Build history of the part. All positions in model axes, mm. Coordinates: 2 decimals unless noted, no trailing zeros. Loops run counter-clockwise (first coordinate to the right, second up) from the corner with the lowest first, then second, coordinate; pieces in that order, holes last. Notation, with made-up numbers: (84, -3) - (99, -3) arc R17 cw to (99, 4) - close; hole circle Ø4 at (62, 82.25). An arc over 180 degrees is marked (long way). One line per item, written item: value.
```python
from build123d import *

# Parameters (mm, degrees)
F1_DEPTH = 20
F2_DEPTH = 12
F3_DEPTH = 2
F4_D     = 3.3


with BuildPart() as f1:
    # F0 (on Top) → F1 (new body)
    with BuildSketch(Plane.XY):
        with BuildLine():
            Line((0, 0), (0, 5))
            ThreePointArc((0, 5), (-3.5355339059, -3.5355339059), (5, 0))
            Line((5, 0), (0, 0))
        make_face()
        with BuildLine():
            Line((0, 0), (5, 0))
            ThreePointArc((5, 0), (4.6193976626, 1.9134171618), (3.5355339059, 3.5355339059))
            Line((3.5355339059, 3.5355339059), (0, 0))
        make_face()
        with BuildLine():
            ThreePointArc((3.5355339059, 3.5355339059), (1.9134171618, 4.6193976626), (0, 5))
            Line((0, 5), (0, 0))
            Line((0, 0), (3.5355339059, 3.5355339059))
        make_face()
    extrude(amount=F1_DEPTH)

    # F0 (on Top) → F2 (join)
    with BuildSketch(Plane.XY):
        with BuildLine():
            Line((24.7487373415, 29.7487373415), (0, 5))
            ThreePointArc((0, 5), (1.9134171618, 4.6193976626), (3.5355339059, 3.5355339059))
            ThreePointArc((3.5355339059, 3.5355339059), (4.6193976626, 1.9134171618), (5, 0))
            Line((5, 0), (29.7487373415, 24.7487373415))
            Line((29.7487373415, 24.7487373415), (24.7487373415, 29.7487373415))
        make_face()
    extrude(amount=F2_DEPTH)

    # F0 (on Top) → F3 (cut)
    with BuildSketch(Plane.XY):
        with BuildLine():
            Line((24.7487373415, 29.7487373415), (0, 5))
            ThreePointArc((0, 5), (1.9134171618, 4.6193976626), (3.5355339059, 3.5355339059))
            ThreePointArc((3.5355339059, 3.5355339059), (4.6193976626, 1.9134171618), (5, 0))
            Line((5, 0), (29.7487373415, 24.7487373415))
            Line((29.7487373415, 24.7487373415), (24.7487373415, 29.7487373415))
        make_face()
    extrude(amount=F3_DEPTH, mode=Mode.SUBTRACT)

    # F4 (through all)
    with Locations(Plane(origin=(0, 0, 0), x_dir=(1, 0, 0), z_dir=(0, 0, -1))):
        with Locations((0, 0)):
            Hole(F4_D / 2)


solid = f1.part
```
Item 1: Cut at D-D, the plane x = 15. Write the cut outline in (y, z), then the cut area to 3 significant figures.
Check result:
outline: (10, 2) - (20, 2) - (20, 12) - (10, 12) - close
area: 100 mm^2
Item 2: Probe probe 1 along Y at (x, z) = (0, 8.5); probe 2 along Z at (x, y) = (9.5, 8); probe 3 along X at (y, z) = (1, 10.5). List the from-to ranges inside material, lowest first. Write a range as from..to.
Check result:
probe 1: y = -5..-1.65, 1.65..5
probe 2: z = 2..12
probe 3: x = -4.9..-1.31, 1.31..6
Item 3: Cut at C-C, the plane y = 4. Write the cut outline in (x, z).
Check result:
outline: (-3, 0) - (3, 0) - (3, 2) - (9, 2) - (9, 12) - (3, 12) - (3, 20) - (-3, 20) - close
Item 4: Drop flat-ended pins along their axis: P1, Ø3, axis at x = 11, z = 12.5, coming from the +Y side; P2, Ø8, axis at y = 20.5, z = 4.5, coming from the -X side; P3, Ø6, axis at x = 15.5, y = 6.5, coming from the +Z side. Give the stop position or say it passes through.
Check result:
P1: stops at y = 17.41
P2: stops at x = 11.5
P3: stops at z = 12
Item 5: Pull direction X, two halves, no side cores. Call faces 1 (the face through (0, -2, 20)), 2 (the face through (13, 18, 7)), 3 (the face through (1.216, -1.115, 10.14)): released by +X, released by -X, zero draft, split by the parting line, or undercut.
Check result:
face 1: zero draft
face 2: released by -X
face 3: undercut
Item 6: Cut at B-B, the plane z = 13.25. Write the cut outline in (x, y), then the cut area to 3 significant figures.
Check result:
outline: circle Ø10 at (0, 0); hole circle Ø3.3 at (0, 0)
area: 70.0 mm^2
Item 7: Cut at A-A, the plane x = -1. Write the cut outline in (y, z).
Check result:
outline: (-4.9, 0) - (-1.31, 0) - (-1.31, 20) - (-4.9, 20) - close; (1.31, 0) - (4.9, 0) - (4.9, 20) - (1.31, 20) - close
